from build123d import *

# Parameters (mm, degrees)
SCHIZZO1_W                             = 117.6
SCHIZZO1_H                             = 66.8
ESTRUSIONE_ESTRUSIONE1_DEPTH           = 3
RACCORDO1_R                            = 2
RACCORDO2_R                            = 2
RACCORDO3_R                            = 2
RACCORDO4_R                            = 2
FORO_SVASATO_PER_VITE_M2_1_D           = 2.6
FORO_SVASATO_PER_VITE_M2_1_CSINK_D     = 4.4
FORO_SVASATO_PER_VITE_M2_1_CSINK_ANGLE = 90


with BuildPart() as part:
    # Schizzo1 → Estrusione-Estrusione1 (new body)
    with BuildSketch(Plane.XY):
        Rectangle(SCHIZZO1_W, SCHIZZO1_H)
    extrude(amount=ESTRUSIONE_ESTRUSIONE1_DEPTH)

    # Raccordo1
    raccordo1_edges = [part.edges().sort_by_distance(p)[0] for p in [
        (-58.8, 33.4, 1.5),
    ]]
    fillet(raccordo1_edges, radius=RACCORDO1_R)

    # Raccordo2
    raccordo2_edges = [part.edges().sort_by_distance(p)[0] for p in [
        (58.8, 33.4, 1.5),
    ]]
    fillet(raccordo2_edges, radius=RACCORDO2_R)

    # Raccordo3
    raccordo3_edges = [part.edges().sort_by_distance(p)[0] for p in [
        (58.8, -33.4, 1.5),
    ]]
    fillet(raccordo3_edges, radius=RACCORDO3_R)

    # Raccordo4
    raccordo4_edges = [part.edges().sort_by_distance(p)[0] for p in [
        (-58.8, -33.4, 1.5),
    ]]
    fillet(raccordo4_edges, radius=RACCORDO4_R)

    # Foro svasato per Vite M2-1 (through all)
    with Locations(Plane.XY.offset(3)):
        with Locations((53.5, 28.1), (-53.5, 28.1), (-53.5, -28.1), (53.5, -28.1)):
            CounterSinkHole(FORO_SVASATO_PER_VITE_M2_1_D / 2, FORO_SVASATO_PER_VITE_M2_1_CSINK_D / 2, counter_sink_angle=FORO_SVASATO_PER_VITE_M2_1_CSINK_ANGLE)


solid = part.part
CAD build for the part. Positions are in the model's coordinates, mm. Round coordinates to 2 decimals unless told otherwise and drop trailing zeros. Write each loop counter-clockwise with the first axis right and the second up, starting at its lowest first coordinate (ties: lowest second). Pieces come first, ordered by that corner, then holes. Notation, with made-up numbers: M 2.5,46.5 L 11.5,46.5 A13 cw 11.5,53.5 Z; hole C 50.25,13 d8. An arc over 180 degrees is marked long. Use a Markdown table: item, result. Add a question column.
1. Slice it at B-B on x = 53.5. Give the cut face in (y, z), then the cut area to 3 significant figures.
2. Pull direction X, two halves, no side cores. Call faces 1 (the face through (52.9, 26.947, 1.035)), 2 (the face through (58.8, 0, 1)), 3 (the face through (-1, 0, 3)): released by +X, released by -X, zero draft, split by the parting line, or undercut.
3. Slice it at A-A on y = -28.1. Give the cut face in (x, z).
4. Drill centre lines: probe 1 along X at (y, z) = (-28, 1.35); probe 2 along Y at (x, z) = (-53.5, 0.8); probe 3 along Y at (x, z) = (-53, 2.6). Where is each one in solid material? Low to high.
5. Flat gauge pin, fed straight in: P1, Ø2, axis at x = -53.5, y = -28.1, coming from the +Z side. Where does the tip first touch, or does it go through?
Reply:
| question | item | result |
|---|---|---|
| 1 | outline | M -33.4,0 L -29.4,0 L -29.4,2.1 L -30.3,3 L -33.4,3 Z; M -26.8,0 L 26.8,0 L 26.8,2.1 L 25.9,3 L -25.9,3 L -26.8,2.1 Z; M 29.4,0 L 33.4,0 L 33.4,3 L 30.3,3 L 29.4,2.1 Z |
| 1 | area | 183 mm^2 |
| 2 | face 1 | undercut |
| 2 | face 2 | released by +X |
| 2 | face 3 | zero draft |
| 3 | outline | M -58.8,0 L -54.8,0 L -54.8,2.1 L -55.7,3 L -58.8,3 Z; M -52.2,0 L 52.2,0 L 52.2,2.1 L 51.3,3 L -51.3,3 L -52.2,2.1 Z; M 54.8,0 L 58.8,0 L 58.8,3 L 55.7,3 L 54.8,2.1 Z |
| 4 | probe 1 | x = -58.8 to -54.8, -52.2 to 52.2, 54.8 to 58.8 |
| 4 | probe 2 | y = -33.4 to -29.4, -26.8 to 26.8, 29.4 to 33.4 |
| 4 | probe 3 | y = -33.4 to -29.83, -26.37 to 26.37, 29.83 to 33.4 |
| 5 | P1 | passes through |
